from build123d import *

# Parameters (mm, degrees)
SKETCH1_W           = 105
SKETCH1_H           = 105
BOSS_EXTRUDE1_DEPTH = 38
SKETCH2_W           = 97
SKETCH2_H           = 97
CUT_EXTRUDE1_DEPTH  = 34
SKETCH3_W           = 101
SKETCH3_H           = 101
CUT_EXTRUDE2_DEPTH  = 8
SKETCH5_R           = 1.6
CUT_EXTRUDE3_DEPTH  = 106
CUT_EXTRUDE4_REACH  = 6
SKETCH7_R           = 8.1
CUT_EXTRUDE5_DEPTH  = 1
SKETCH11_R          = 1.3
CUT_EXTRUDE6_DEPTH  = 106
CUT_EXTRUDE7_REACH  = 107
SKETCH12_R          = 1.55


with BuildPart() as part:
    # Sketch1 → Boss-Extrude1 (new body)
    with BuildSketch(Plane(origin=(0, 0, 0), x_dir=(1, 0, 0), z_dir=(0, 1, 0))):
        Rectangle(SKETCH1_W, SKETCH1_H)
    extrude(amount=BOSS_EXTRUDE1_DEPTH)

    # Sketch2 → Cut-Extrude1 (cut)
    with BuildSketch(Plane(origin=(0, 38, 0), x_dir=(1, 0, 0), z_dir=(0, 1, 0))):
        Rectangle(SKETCH2_W, SKETCH2_H)
    extrude(amount=-CUT_EXTRUDE1_DEPTH, mode=Mode.SUBTRACT)

    # Sketch3 → Cut-Extrude2 (cut)
    with BuildSketch(Plane(origin=(0, 38, 0), x_dir=(1, 0, 0), z_dir=(0, 1, 0))):
        Rectangle(SKETCH3_W, SKETCH3_H)
    extrude(amount=-CUT_EXTRUDE2_DEPTH, mode=Mode.SUBTRACT)

    # Sketch5 → Cut-Extrude3 (cut, through all)
    with BuildSketch(Plane(origin=(52.5, 0, 0), x_dir=(0, 0, -1), z_dir=(1, 0, 0))):
        with Locations((0, 34)):
            Circle(SKETCH5_R)
    extrude(amount=-CUT_EXTRUDE3_DEPTH, mode=Mode.SUBTRACT)

    # Sketch7 → Cut-Extrude4 (cut, up to next)
    with BuildSketch(Plane(origin=(0, 0, 48.5), x_dir=(-1, 0, 0), z_dir=(0, 0, -1)), mode=Mode.PRIVATE) as cut_extrude4_sk1:
        with Locations((0, 18)):
            Circle(SKETCH7_R)
    cut_extrude4_tool1 = extrude(cut_extrude4_sk1.sketch, amount=-CUT_EXTRUDE4_REACH, mode=Mode.PRIVATE) & part.part
    add(cut_extrude4_tool1.solids().sort_by_distance((0, 18, 48.5))[0], mode=Mode.SUBTRACT)

    # Sketch10 → Cut-Extrude5 (cut)
    with BuildSketch(Plane.XZ):
        with BuildLine():
            Line((5, -10), (0, -10))
            ThreePointArc((0, -10), (-5, -5), (0, 0))
            ThreePointArc((0, 0), (-5, 5), (0, 10))
            Line((0, 10), (5, 10))
            Line((5, 10), (5, -10))
        make_face()
        with BuildLine():
            Line((0, -7), (2, -7))
            Line((2, -7), (2, -3))
            Line((2, -3), (0, -3))
            ThreePointArc((0, -3), (-2, -5), (0, -7))
        make_face(mode=Mode.SUBTRACT)
        with BuildLine():
            Line((0, 3), (2, 3))
            Line((2, 3), (2, 7))
            Line((2, 7), (0, 7))
            ThreePointArc((0, 7), (-2, 5), (0, 3))
        make_face(mode=Mode.SUBTRACT)
    extrude(amount=-CUT_EXTRUDE5_DEPTH, mode=Mode.SUBTRACT)

    # Sketch11 → Cut-Extrude6 (cut, through all)
    with BuildSketch(Plane.XY.offset(52.5)):
        with Locations((-37.5, 22)):
            Circle(SKETCH11_R)
        with Locations((37.5, 22)):
            Circle(SKETCH11_R)
    extrude(amount=-CUT_EXTRUDE6_DEPTH, mode=Mode.SUBTRACT)

    # Sketch12 → Cut-Extrude7 (cut, up to next)
    with BuildSketch(Plane(origin=(0, 0, -52.5), x_dir=(-1, 0, 0), z_dir=(0, 0, -1)), mode=Mode.PRIVATE) as cut_extrude7_sk1:
        with Locations((0, 10)):
            Circle(SKETCH12_R)
    cut_extrude7_tool1 = extrude(cut_extrude7_sk1.sketch, amount=-CUT_EXTRUDE7_REACH, mode=Mode.PRIVATE) & part.part
    add(cut_extrude7_tool1.solids().sort_by_distance((0, 10, -52.5))[0], mode=Mode.SUBTRACT)


solid = part.part
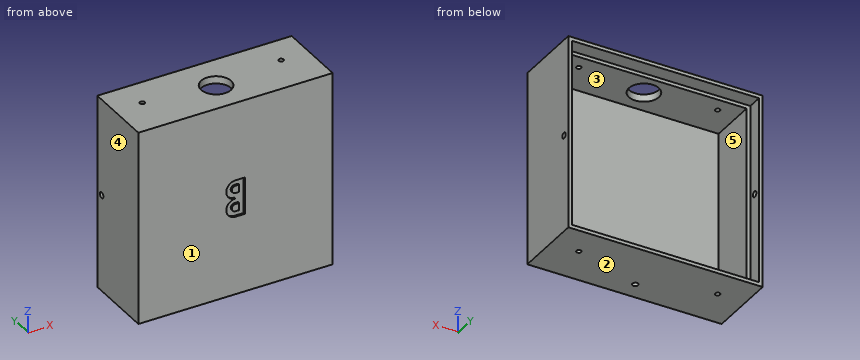
Could you check a few things on this model? Use its own coordinates, in mm. Face numbers are marked on the shaded views. A direction names the side the tool comes from. Give positions to 0.01 mm unless a question says otherwise; leave off trailing zeros. Write each loop counter-clockwise with the first axis right and the second up, starting at its lowest first coordinate (ties: lowest second). Pieces come first, ordered by that corner, then holes. Notation, with made-up numbers: (50, 25) - (66, 25) arc R20 cw to (66, 45) - close; hole circle Ø9 at (-4.75, 19). An arc over 180 degrees is marked (long way). Use CSV: the item, a comma, the result in double quotes. Start each with the question number.
Item 1: If we mould it in two halves opening along Z, with no side actions, what happens to the marked faces 1, 2 and 3? For each: pulls with the +Z half, pulls with the -Z half, needs draft (parallel to the pull), parting line crosses it, or undercut.
Item 2: I want a section at B-B, the plane y = 34. Please give me the cut outline in (x, z), then the cut area to 3 significant figures.
Item 3: I want a section at C-C, the plane y = 22. Please give me the cut outline in (x, z), then the cut area to 3 significant figures.
Item 4: I want a section at A-A, the plane x = 37.5. Please give me the cut outline in (y, z), then the cut area to 3 significant figures.
Item 5: I want a section at D-D, the plane z = 12. Please give me the cut outline in (x, y).
Item 6: For the marked faces 4 and 5, which set-ups out of +Z, -Z, +X, -X, +Y, -Y let a thin tool reach every point of the face, with its end or its side?
Item 7: If I drill on line 1 along Y through (x, z) = (37.5, 51.1); line 2 along X through (y, z) = (13, 39); line 3 along Z through (x, y) = (-41, 32.5), over which ranges is the centre line in solid material (lowest first)?
Item 8: I'm going to push flat-ended pins straight in: pin 1 (13 mm diameter, centred on x = 0, y = 18, fed in from +Z); pin 2 (8 mm diameter, centred on x = -0.5, z = 3.5, fed in from -Y). Where does each tip first touch, or does it pass through?
Findings:
1,face 1,"needs draft"
1,face 2,"pulls with the -Z half"
1,face 3,"undercut"
2,outline,"(-52.5, -52.5) - (52.5, -52.5) - (52.5, -1.6) - (50.5, -1.6) - (50.5, -50.5) - (-50.5, -50.5) - (-50.5, -1.6) - (-52.5, -1.6) - close; (-52.5, 1.6) - (-50.5, 1.6) - (-50.5, 50.5) - (50.5, 50.5) - (50.5, 1.6) - (52.5, 1.6) - (52.5, 52.5) - (-52.5, 52.5) - close"
2,area,"811 mm2"
3,outline,"(-52.5, -52.5) - (-38.8, -52.5) - (-38.8, -48.5) - (-48.5, -48.5) - (-48.5, 48.5) - (-38.8, 48.5) - (-38.8, 52.5) - (-52.5, 52.5) - close; (-36.2, -52.5) - (36.2, -52.5) - (36.2, -48.5) - (-36.2, -48.5) - close; (-36.2, 48.5) - (-7.04, 48.5) - (-7.04, 52.5) - (-36.2, 52.5) - close; (7.04, 48.5) - (36.2, 48.5) - (36.2, 52.5) - (7.04, 52.5) - close; (38.8, -52.5) - (52.5, -52.5) - (52.5, 52.5) - (38.8, 52.5) - (38.8, 48.5) - (48.5, 48.5) - (48.5, -48.5) - (38.8, -48.5) - close"
3,area,"1,520 mm2"
4,outline,"(0, -52.5) - (20.7, -52.5) - (20.7, -48.5) - (4, -48.5) - (4, 48.5) - (20.7, 48.5) - (20.7, 52.5) - (0, 52.5) - close; (23.3, -52.5) - (38, -52.5) - (38, -50.5) - (30, -50.5) - (30, -48.5) - (23.3, -48.5) - close; (23.3, 48.5) - (30, 48.5) - (30, 50.5) - (38, 50.5) - (38, 52.5) - (23.3, 52.5) - close"
4,area,"639 mm2"
5,outline,"(-52.5, 0) - (52.5, 0) - (52.5, 38) - (50.5, 38) - (50.5, 30) - (48.5, 30) - (48.5, 4) - (-48.5, 4) - (-48.5, 30) - (-50.5, 30) - (-50.5, 38) - (-52.5, 38) - close"
6,face 4,"+Z, -Z, -X, +Y, -Y"
6,face 5,"+Y"
7,line 1,"y = 0 to 20.7, 23.3 to 38"
7,line 2,"x = -52.5 to -48.5, 48.5 to 52.5"
7,line 3,"z = -52.5 to -50.5, 50.5 to 52.5"
8,pin 1,"stops at z = -48.5"
8,pin 2,"stops at y = 0"
